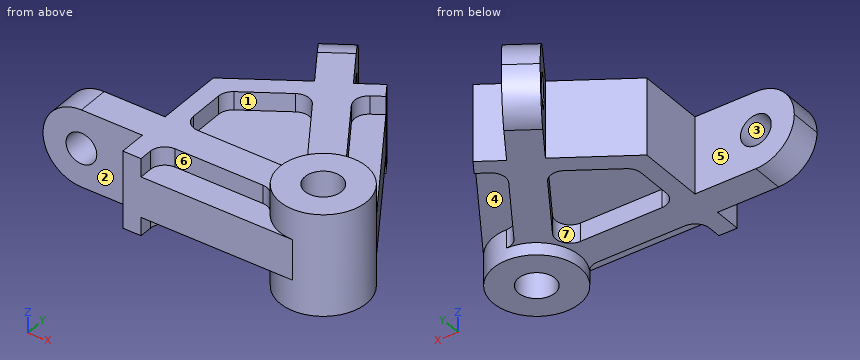
from build123d import *

# Parameters (mm, degrees)
SKETCH1_R               = 22.5
SKETCH1_R_2             = 9.5
BOSS_EXTRUDE1_DEPTH     = 26.35
BOSS_EXTRUDE2_DEPTH     = 20
BOSS_EXTRUDE3_DEPTH     = 10.5
CUT_EXTRUDE1_DEPTH      = 180.896655326
CUT_EXTRUDE1_DEPTH_BACK = 180.896655326
SKETCH2_R               = 8
CUT_EXTRUDE2_DEPTH      = 183.770827506
CUT_EXTRUDE2_DEPTH_BACK = 183.770827506


with BuildPart() as part:
    # Sketch1 → Boss-Extrude1 (new, symmetric)
    with BuildSketch(Plane.XY):
        with Locations(Location((0, 0, 0), (0, 0, 180))):
            Circle(SKETCH1_R)
        with Locations(Location((0, 0, 0), (0, 0, 180))):
            Circle(SKETCH1_R_2, mode=Mode.SUBTRACT)
    extrude(amount=BOSS_EXTRUDE1_DEPTH, both=True)

    # Sketch1_3 → Boss-Extrude2 (add, symmetric)
    with BuildSketch(Plane.XY):
        with BuildLine():
            Line((-26.688113545, 71.205201109), (-20.995221285, 74.831973466))
            Line((-20.995221285, 74.831973466), (-25.685065162, 82.193553759))
            Line((-25.685065162, 82.193553759), (-37.703393265, 74.53703434))
            Line((-37.703393265, 74.53703434), (-60.204471615, 109.856652495))
            Line((-60.204471615, 109.856652495), (-74.120430471, 100.991208958))
            Line((-74.120430471, 100.991208958), (-52.033854523, 66.322229244))
            Line((-52.033854523, 66.322229244), (-88.25, 43.25))
            Line((-88.25, 43.25), (-88.25, 8.25))
            Line((-88.25, 8.25), (-140, 8.25))
            Line((-140, 8.25), (-140, -8.25))
            Line((-140, -8.25), (-88.25, -8.25))
            Line((-88.25, -8.25), (-88.25, -22.5))
            Line((-88.25, -22.5), (-78.75, -22.5))
            Line((-78.75, -22.5), (-78.75, -15.75))
            ThreePointArc((-78.75, -15.75), (-76.553300859, -10.446699141), (-71.25, -8.25))
            Line((-71.25, -8.25), (-25.533066796, -8.25))
            ThreePointArc((-25.533066796, -8.25), (-21.878018917, -9.200906551), (-19.149800097, -11.8125))
            ThreePointArc((-19.149800097, -11.8125), (-19.726352003, 10.822247301), (-0.326618638, 22.497629214))
            ThreePointArc((-0.326618638, 22.497629214), (-3.995085116, 23.395377492), (-6.760927361, 25.96709189))
            Line((-6.760927361, 25.96709189), (-28.983802326, 60.850018203))
            ThreePointArc((-28.983802326, 60.850018203), (-29.980586535, 66.50306237), (-26.688113545, 71.205201109))
        make_face()
        with BuildLine():
            ThreePointArc((-53.254944088, 54.280263446), (-47.60189992, 55.277047656), (-42.899761181, 51.984574665))
            Line((-42.899761181, 51.984574665), (-22.383023261, 19.779747063))
            ThreePointArc((-22.383023261, 19.779747063), (-22.133008437, 12.142584233), (-28.708459105, 8.25))
            Line((-28.708459105, 8.25), (-71.25, 8.25))
            ThreePointArc((-71.25, 8.25), (-76.553300859, 10.446699141), (-78.75, 15.75))
            Line((-78.75, 15.75), (-78.75, 33.923480627))
            ThreePointArc((-78.75, 33.923480627), (-77.825450668, 37.530896394), (-75.279747063, 40.248916471))
            Line((-75.279747063, 40.248916471), (-53.254944088, 54.280263446))
        make_face(mode=Mode.SUBTRACT)
    extrude(amount=BOSS_EXTRUDE2_DEPTH, both=True)

    # Sketch1_4 → Boss-Extrude3 (add, symmetric)
    with BuildSketch(Plane.XY):
        with BuildLine():
            ThreePointArc((-71.25, 8.25), (-76.553300859, 10.446699141), (-78.75, 15.75))
            Line((-78.75, 15.75), (-78.75, 33.923480627))
            ThreePointArc((-78.75, 33.923480627), (-77.825450668, 37.530896394), (-75.279747063, 40.248916471))
            Line((-75.279747063, 40.248916471), (-53.254944088, 54.280263446))
            ThreePointArc((-53.254944088, 54.280263446), (-47.60189992, 55.277047656), (-42.899761181, 51.984574665))
            Line((-42.899761181, 51.984574665), (-22.383023261, 19.779747063))
            ThreePointArc((-22.383023261, 19.779747063), (-22.133008437, 12.142584233), (-28.708459105, 8.25))
            Line((-28.708459105, 8.25), (-71.25, 8.25))
        make_face()
        with BuildLine():
            ThreePointArc((-0.326618638, 22.497629214), (10.678780795, 19.804384381), (18.976307531, 12.089241188))
            Line((18.976307531, 12.089241188), (-20.995221285, 74.831973466))
            Line((-20.995221285, 74.831973466), (-26.688113545, 71.205201109))
            ThreePointArc((-26.688113545, 71.205201109), (-29.980586535, 66.50306237), (-28.983802326, 60.850018203))
            Line((-28.983802326, 60.850018203), (-6.760927361, 25.96709189))
            ThreePointArc((-6.760927361, 25.96709189), (-3.995085116, 23.395377492), (-0.326618638, 22.497629214))
        make_face()
        with BuildLine():
            Line((-78.75, -22.5), (0, -22.5))
            ThreePointArc((0, -22.5), (-10.965143638, -19.647280346), (-19.149800097, -11.8125))
            ThreePointArc((-19.149800097, -11.8125), (-21.878018917, -9.200906551), (-25.533066796, -8.25))
            Line((-25.533066796, -8.25), (-71.25, -8.25))
            ThreePointArc((-71.25, -8.25), (-76.553300859, -10.446699141), (-78.75, -15.75))
            Line((-78.75, -15.75), (-78.75, -22.5))
        make_face()
    extrude(amount=BOSS_EXTRUDE3_DEPTH, both=True)

    # Sketch2 → Cut-Extrude1 (cut, two sides: drawn at the far end of the back side and taken through both)
    with BuildSketch(Plane(origin=(0, 0, 0), x_dir=(1, 0, 0), z_dir=(0, 1, 0)).offset(-CUT_EXTRUDE1_DEPTH_BACK)):
        with BuildLine():
            Line((-140, -20), (-120, -20))
            ThreePointArc((-120, -20), (-134.142135662, -14.142135586), (-140, 1.08e-07))
            Line((-140, 1.08e-07), (-140, -20))
        make_face()
        with BuildLine():
            ThreePointArc((-140, 1.08e-07), (-134.142135586, 14.142135662), (-120, 20))
            Line((-120, 20), (-140, 20))
            Line((-140, 20), (-140, 1.08e-07))
        make_face()
        with Locations(Location((-120, 0, 0), (0, 0, 270))):
            Circle(SKETCH2_R)
    extrude(amount=CUT_EXTRUDE1_DEPTH + CUT_EXTRUDE1_DEPTH_BACK, mode=Mode.SUBTRACT)

    # Sketch4 → Cut-Extrude2 (cut, two sides: drawn at the far end of the back side and taken through both)
    with BuildSketch(Plane(origin=(6.957979428, 4.432721769, 0), x_dir=(0, 0, -1), z_dir=(0.8433914458128867, 0.5372996083468223, 0)).offset(-CUT_EXTRUDE2_DEPTH_BACK)):
        with BuildLine():
            ThreePointArc((-4.3e-08, 125), (14.142135608, 119.142135639), (20, 105))
            Line((20, 105), (20, 125))
            Line((20, 125), (-4.3e-08, 125))
        make_face()
        with BuildLine():
            ThreePointArc((-20, 105), (-14.142135639, 119.142135608), (-4.3e-08, 125))
            Line((-4.3e-08, 125), (-20, 125))
            Line((-20, 125), (-20, 105))
        make_face()
        with BuildLine():
            ThreePointArc((0, 113), (-8, 105), (0, 97))
            Line((0, 97), (0, 113))
        make_face()
        with BuildLine():
            Line((0, 113), (0, 97))
            ThreePointArc((0, 97), (5.656854249, 99.343145751), (8, 105))
            ThreePointArc((8, 105), (5.656854249, 110.656854249), (0, 113))
        make_face()
    extrude(amount=CUT_EXTRUDE2_DEPTH + CUT_EXTRUDE2_DEPTH_BACK, mode=Mode.SUBTRACT)


solid = part.part
Geometry: final body of the model. Coordinates: model frame, mm. Face numbers are marked on the shaded views. A direction names the side the tool comes from. Round coordinates to 2 decimals unless told otherwise and drop trailing zeros. Write each loop counter-clockwise with the first axis right and the second up, starting at its lowest first coordinate (ties: lowest second). Pieces come first, ordered by that corner, then holes. Notation, with made-up numbers: M -24,18.25 L 25,18.25 A22 cw 25,55.25 Z; hole C 26,39.25 d8. An arc over 180 degrees is marked long. Write item = value, one per line.
Item 1: Section query A-A on y = 0. Return loops of the section in (x, z).
Findings:
outline = M -120,-20 L -22.5,-20 L -22.5,-26.35 L -9.5,-26.35 L -9.5,26.35 L -22.5,26.35 L -22.5,20 L -120,20 A20 ccw Z; M 9.5,-26.35 L 22.5,-26.35 L 22.5,26.35 L 9.5,26.35 Z; hole C -120,0 d16
Item 2: Pin query (flat end, axial travel): P1, Ø10, axis at y = 30.5, z = 14.5, coming from the +X side; P2, Ø5, axis at y = 63.5, z = -9, coming from the +X side; P3, Ø18.5, axis at x = -120, z = 0, coming from the +Y side. Return the tip coordinate at first contact, or that it passes through.
Findings:
P1 = 9.16
P2 = -12.18
P3 = 8.25
Item 3: Section query C-C on x = -123. Return loops of the section in (y, z).
Findings:
outline = M -8.25,-19.77 L 8.25,-19.77 L 8.25,-7.42 L -8.25,-7.42 Z; M -8.25,7.42 L 8.25,7.42 L 8.25,19.77 L -8.25,19.77 Z
Item 4: Section query B-B on z = -4. Return loops of the section in (x, y), then the cut area to 3 significant figures.
Findings:
outline = M -139.6,-8.25 L -126.93,-8.25 L -126.93,8.25 L -139.6,8.25 Z; M -113.07,-8.25 L -88.25,-8.25 L -88.25,-22.5 L 0,-22.5 A22.5 ccw 18.98,12.09 L -25.69,82.19 L -37.7,74.54 L -45.74,87.15 L -59.65,78.28 L -52.03,66.32 L -88.25,43.25 L -88.25,8.25 L -113.07,8.25 Z; M -73.9,100.65 L -67.1,89.97 L -53.18,98.83 L -59.99,109.52 Z; hole C 0,0 d19
area = 9,240 mm^2
Item 5: Pull-direction query (Y, two-part tool) for the marked faces 1, 2 and 3; classes: pulls with the +Y half, pulls with the -Y half, needs draft (parallel to the pull), parting line crosses it, or undercut.
Findings:
face_1 = undercut
face_2 = pulls with the -Y half
face_3 = needs draft
Item 6: Access query for the marked faces 4, 5, 6 and 7. Directions: +Z, -Z, +X, -X, +Y, -Y. A direction counts if a zero-diameter tool reaches every point of the face in a straight line with its end or side. Return the directions, or none.
Findings:
face_4 = -Z, +X
face_5 = +Z, -Z, -X, +Y
face_6 = +Z, -Y
face_7 = -Z
Item 7: Material intervals for line 1 along Y through (x, z) = (0, 15.5); line 2 along Z through (x, y) = (-69, 16); line 3 along X through (y, z) = (3, 0), sorted ascending. Write a range as [from, to].
Findings:
line_1 = [-22.5, -9.5], [9.5, 22.5]
line_2 = [-10.5, 10.5]
line_3 = [-140, -128], [-112, -9.01], [9.01, 22.3]
Item 8: Section query D-D on z = 22. Return loops of the section in (x, y).
Findings:
outline = C 0,0 d45; hole C 0,0 d19
